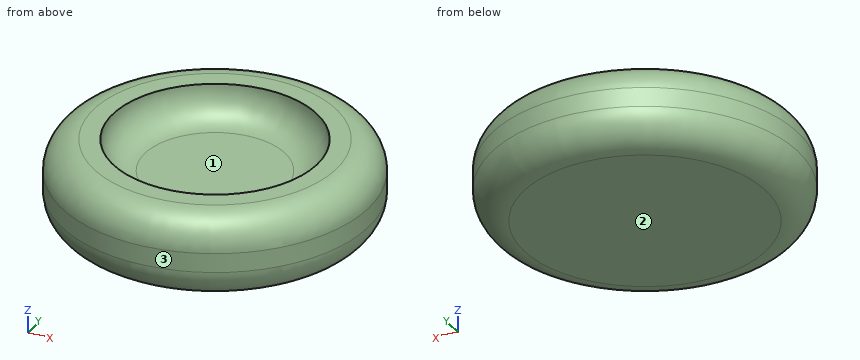
from build123d import *

# Parameters (mm, degrees)
F0_R     = 16
F1_DEPTH = 5
F2_T     = 8


# Not quite as in the source:
# - a fillet or chamfer that OpenCascade refuses, or shapes differently, is made with other operations: its cross-section is extruded or revolved along the edge and cut away or added
# - two fillets or chamfers of one size are made in one step
# - a feature of the source that left no trace in its solid (it failed there, or was rolled back) is left out


with BuildPart() as f1:
    # F0 (on Top) → F1 (new body)
    with BuildSketch(Plane.XY):
        with Locations((-3.0124252662, 6.3863405958)):
            Circle(F0_R)
    extrude(amount=F1_DEPTH)

    # F2
    f2_openings = [f1.faces().sort_by_distance(p)[0] for p in [
        (-3.012425, 6.386341, 5),
    ]]
    offset(amount=F2_T, openings=f2_openings, kind=Kind.INTERSECTION)

    # F3: fillet of radius 5 on 3 edges, made by hand

    # F3_s1 → F3_t2 (revolve)
    with BuildSketch(Plane.XZ.offset(-6.3863405958)):
        with BuildLine():
            ThreePointArc((12.9875747338, 5), (11.5231086397, 1.4644660941), (7.9875747338, 0))
            Line((7.9875747338, 0), (12.9875747338, 0))
            Line((12.9875747338, 0), (12.9875747338, 5))
        make_face()
    revolve(axis=Axis((-3.0124252662, 6.3863405958, 0), (0, 0, 1)))

    # F3_s3 → F3_t4 (revolve, cut)
    with BuildSketch(Plane.XZ.offset(-6.3863405958)):
        with BuildLine():
            ThreePointArc((15.9875747338, 5), (19.5231086397, 3.5355339059), (20.9875747338, 0))
            Line((20.9875747338, 0), (20.9875747338, 5))
            Line((20.9875747338, 5), (15.9875747338, 5))
        make_face()
    revolve(axis=Axis((-3.0124252662, 6.3863405958, 5), (0, 0, -1)), mode=Mode.SUBTRACT)

    # F3_s5 → F3_t6 (revolve, cut)
    with BuildSketch(Plane.XZ.offset(-6.3863405958)):
        with BuildLine():
            ThreePointArc((20.9875747338, -3), (19.5231086397, -6.5355339059), (15.9875747338, -8))
            Line((15.9875747338, -8), (20.9875747338, -8))
            Line((20.9875747338, -8), (20.9875747338, -3))
        make_face()
    revolve(axis=Axis((-3.0124252662, 6.3863405958, -8), (0, 0, -1)), mode=Mode.SUBTRACT)


solid = f1.part
Verification items for the finished model (mm, model axes). Face numbers are marked on the shaded views. Coordinates: 2 decimals unless noted, no trailing zeros. Loops run counter-clockwise (first coordinate to the right, second up) from the corner with the lowest first, then second, coordinate; pieces in that order, holes last. Notation, with made-up numbers: (79.25, -6) -> (100.25, -6) arc R17 cw to (100.25, 1) -> close; hole circle Ø8 at (40, 67). An arc over 180 degrees is marked (long way). Answer as a JSON object with one key per item and string values. Group by question number.
Item 1: Sectioned sample at A-A on z = -6. Record the boundary of the cut face in (x, y), plus the area to 3 significant figures.
Item 2: Mould release check, pull along Y, two halves, no side actions. Record for the marked faces 1, 2 and 3: +Y half, -Y half, draft (parallel to the pull), parting line (faces both ways), or undercut.
Item 3: Sectioned sample at B-B on z = 4. Record the boundary of the cut face in (x, y), plus the area to 3 significant figures.
Item 4: Sectioned sample at C-C on z = -1.25. Record the boundary of the cut face in (x, y).
Item 5: Scan lines: probe 1 along Z at (x, y) = (1, 12); probe 2 along X at (y, z) = (-4, 3.5); probe 3 along X at (y, z) = (4.5, 2.25). Record each from-to range of solid material in increasing order.
Item 6: Depth check by flat-ended pin: pin 1 (4 mm diameter, centred on x = -3, z = 3, fed in from +Y); pin 2 (5 mm diameter, centred on y = 15.5, z = -6.5, fed in from +X); pin 3 (3 mm diameter, centred on x = 11.5, z = -6, fed in from +Y). Enter the tip coordinate at first touch or a pass-through.
Evaluation:
{
 "1": {"outline": "circle Ø46 at (-3.01, 6.39)", "area": "1,660 mm²"},
 "2": {"face 1": "undercut", "face 2": "draft", "face 3": "parting line"},
 "3": {"outline": "circle Ø44 at (-3.01, 6.39); hole circle Ø31.8 at (-3.01, 6.39)", "area": "726 mm²"},
 "4": {"outline": "circle Ø48 at (-3.01, 6.39)"},
 "5": {"probe 1": "z = -8 to 0", "probe 2": "x = -23.05 to -14.88, 8.85 to 17.03", "probe 3": "x = -26.4 to -18.07, 12.05 to 20.38"},
 "6": {"pin 1": "stops at y = 30.29", "pin 2": "stops at x = 19.51", "pin 3": "stops at y = 25.8"}
}
